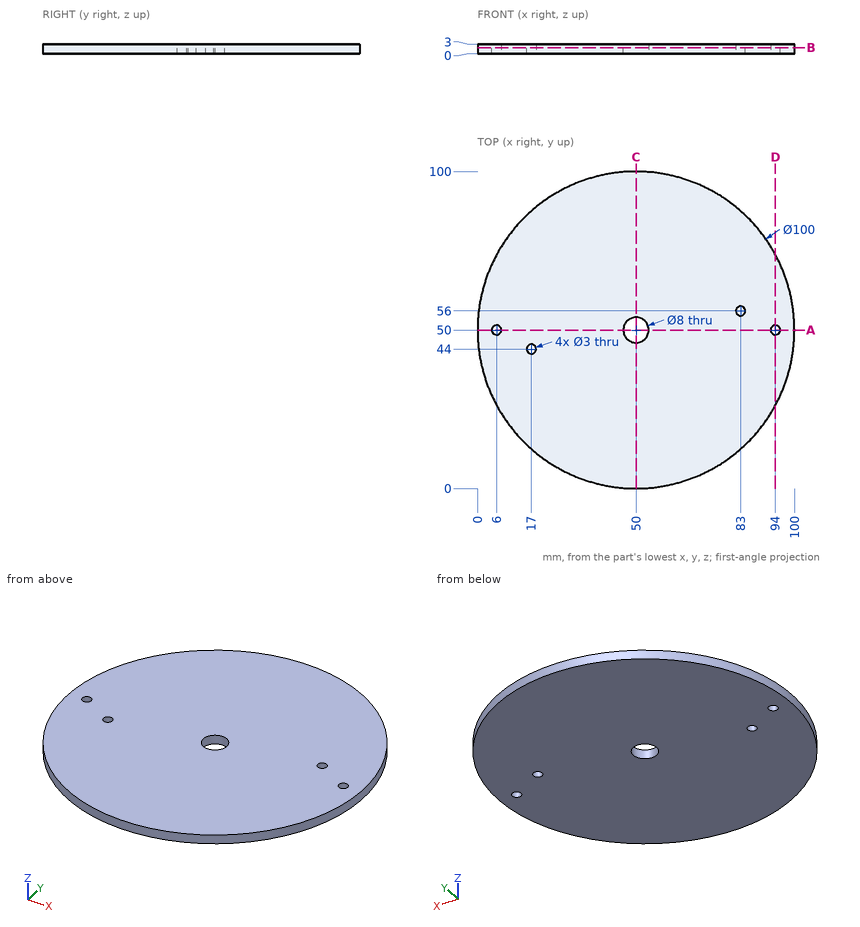
Can you work these out from the drawing? Everything is in mm from the part's minimum corner. Coordinates: 2 decimals unless noted, no trailing zeros. Write each loop counter-clockwise with the first axis right and the second up, starting at its lowest first coordinate (ties: lowest second). Pieces come first, ordered by that corner, then holes. Notation, with made-up numbers: (64, -3.75) -> (104, -3.75) arc R17 cw to (104, 9.25) -> close; hole circle Ø10 at (41.25, 2.25). An arc over 180 degrees is marked (long way). Write each question's results on one line, items separated by ' | '. Start each with the question number.
Item 1: I'm going to push flat-ended pins straight in: P1, Ø1, axis at y = 26.5, z = 1, coming from the -X side; P2, Ø1, axis at x = 49, z = 2, coming from the +Y side. Where does each tip first touch, or does it pass through?
Item 2: If we section it at C-C, the plane x = 50: Write out the boundary of the cut face in (y, z), and give its area (3 significant figures).
Item 3: If we section it at B-B, the plane z = 1.85: Write out the boundary of the cut face in (x, y).
Item 4: If we section it at A-A, the plane y = 50: Write out the boundary of the cut face in (x, z).
Item 5: Please list where these lines run through material, in increasing order: probe 1 along Y at (x, z) = (50, 0.65); probe 2 along Y at (x, z) = (17, 1.45); probe 3 along X at (y, z) = (56, 0.8).
Item 6: If we section it at D-D, the plane x = 94: Write out the boundary of the cut face in (y, z).
Answer block:
1) P1: x = 5.6 | P2: y = 100
2) outline: (0, 0) -> (46, 0) -> (46, 3) -> (0, 3) -> close; (54, 0) -> (100, 0) -> (100, 3) -> (54, 3) -> close | area: 276 mm²
3) outline: circle Ø100 at (50, 50); hole circle Ø3 at (6, 50); hole circle Ø3 at (17, 44); hole circle Ø8 at (50, 50); hole circle Ø3 at (83, 56); hole circle Ø3 at (94, 50)
4) outline: (0, 0) -> (4.5, 0) -> (4.5, 3) -> (0, 3) -> close; (7.5, 0) -> (46, 0) -> (46, 3) -> (7.5, 3) -> close; (54, 0) -> (92.5, 0) -> (92.5, 3) -> (54, 3) -> close; (95.5, 0) -> (100, 0) -> (100, 3) -> (95.5, 3) -> close
5) probe 1: 0 to 46, 54 to 100 | probe 2: 12.44 to 42.5, 45.5 to 87.56 | probe 3: 0.36 to 81.5, 84.5 to 99.64
6) outline: (26.25, 0) -> (48.5, 0) -> (48.5, 3) -> (26.25, 3) -> close; (51.5, 0) -> (73.75, 0) -> (73.75, 3) -> (51.5, 3) -> close
